Autodesk Inventor part; units mm, degrees
ref_plane "YZ Plane" through (0, 0, 0) normal (1, 0, 0) x (0, 1, 0)
ref_plane "XZ Plane" through (0, 0, 0) normal (0, 1, 0) x (-1, 0, 0)
ref_plane "XY Plane" through (0, 0, 0) normal (0, 0, 1) x (1, 0, 0)
sketch "Эскиз1" plane through (0, 0, 0) normal (0, 0, 1) x (1, 0, 0)
  line L0 (0, 0) -> (48, 0) construction
  line L1 (0, -10) -> (48, -10)
  line L2 (48, 10) -> (0, 10)
  arc A0 (0, 10) -> (0, -10) centre (0, 0) ccw
  arc A1 (48, -10) -> (48, 10) centre (48, 0) ccw
  circle A2 centre (0, 0) radius 2.8
  circle A3 centre (48, 0) radius 2.8
  point P0 (24, 0)
  dimension "d0" = 48
  dimension "d1" = 20
  dimension "d2" = 5.6
  dimension "d3" = 5.6
extrude "Выдавливание1" add sketch "Эскиз1" along normal blind 7
chamfer "Фаска1" distance 2 angle 45 2 edges at (-2.8, 0, 0) (45.2, 0, 0)
chamfer "Фаска2" distance 3.5 angle 45 4 edges at (24, 10, 0) (-10, 0, 0) (24, -10, 0) (58, 0, 0)
sketch "Эскиз3" plane through (0, 0, 7) normal (0, 0, 1) x (1, 0, 0)
  circle A0 centre (0, 0) radius 5
  circle A1 centre (48, 0) radius 5
  circle A2 centre (0, 0) radius 2.8
  circle A3 centre (48, 0) radius 2.8
  dimension "d19" = 10
extrude "Выдавливание3" add sketch "Эскиз3" along normal blind 1
chamfer "Фаска4" distance 1 angle 45 6 edges at (24, 10, 7) (-10, 0, 7) (24, -10, 7) (58, 0, 7) (43, 0, 7) (-5, 0, 7)
sketch "Эскиз4" plane through (0, 0, 8) normal (0, 0, 1) x (1, 0, 0)
  circle A0 centre (0, 0) radius 4
  circle A1 centre (48, 0) radius 2.8
  circle A2 centre (48, 0) radius 4
  dimension "d26" = 8
extrude "Выдавливание4" cut sketch "Эскиз4" against normal blind 3.5 contours A0 | A1 | A2
properties part number "Распорка роликов натяжителя"
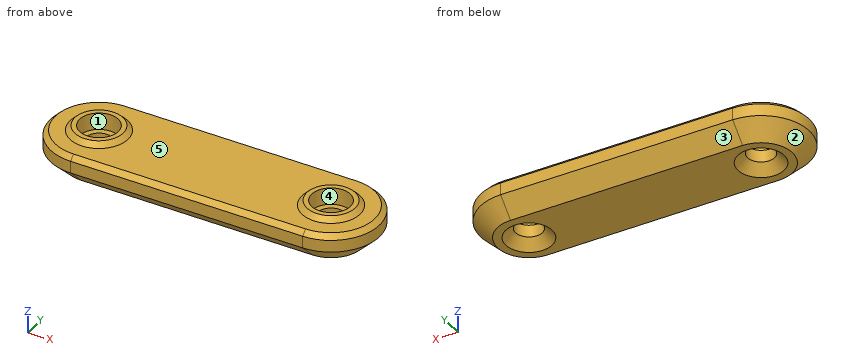
Here's how the part is built. I have some questions about the finished solid (model axes, mm). Face numbers are marked on the shaded views. A direction names the side the tool comes from. Give positions to 0.01 mm unless a question says otherwise; leave off trailing zeros. Order: outer loops, then holes, each group sorted by start corner. A loop starts at its lowest first (then second) coordinate and runs counter-clockwise, first axis right, second up. Notation, with made-up numbers: (30, 76) -> (37, 76) arc R31 ccw to (37, 115) -> close; hole circle Ø1 at (-37.75, -14). An arc over 180 degrees is marked (long way). One line per item, written item: value. Start each with the question number.
1. Imagine slicing it at B-B, the plane y = -1.75. Count the separate pieces of the cut face and the enclosed holes in it, plus the area to 3 significant figures.
2. Will these pins go through, and if not, where does the flat tip stop? pin 1 Ø3 at (y, z) = (7, 1.5) entering from -X; pin 2 Ø1.5 at (x, y) = (40.5, 3.5) entering from +Z; pin 3 Ø9 at (x, y) = (48, 0) entering from -Z.
3. I need wall thicknesses on probe 1 along X at (y, z) = (0, 3.9); probe 2 along X at (y, z) = (0, 2.7); probe 3 along Y at (x, z) = (0, 5.5). Which ranges of each line are inside material? Lowest first, please. Write a range as from..to.
4. We'd pull the mould along Y, two halves only. Please class the marked faces 3, 4 and 5: released by +Y, released by -Y, zero draft, split by the parting line, or undercut.
5. For the marked faces 1 and 2, which set-ups out of +Z, -Z, +X, -X, +Y, -Y let a thin tool reach every point of the face, with its end or its side?
6. Imagine slicing it at A-A, the plane x = 17. List the corners of the cut face in (y, z) for me, plus the area to 3 significant figures.
Values follow:
1. separate pieces: 3
1. enclosed holes: 0
1. area: 382 mm2
2. pin 1: stops at x = -6.89
2. pin 2: stops at z = 7
2. pin 3: stops at z = 0.3
3. probe 1: x = -10..-2.8, 2.8..45.2, 50.8..58
3. probe 2: x = -9.2..-2.8, 2.8..45.2, 50.8..57.2
3. probe 3: y = -10..-4, 4..10
4. face 3: released by +Y
4. face 4: undercut
4. face 5: zero draft
5. face 1: +Z
5. face 2: -Z, -X
6. outline: (-10, 3.5) -> (-6.5, 0) -> (6.5, 0) -> (10, 3.5) -> (10, 6) -> (9, 7) -> (-9, 7) -> (-10, 6) -> close
6. area: 127 mm2
